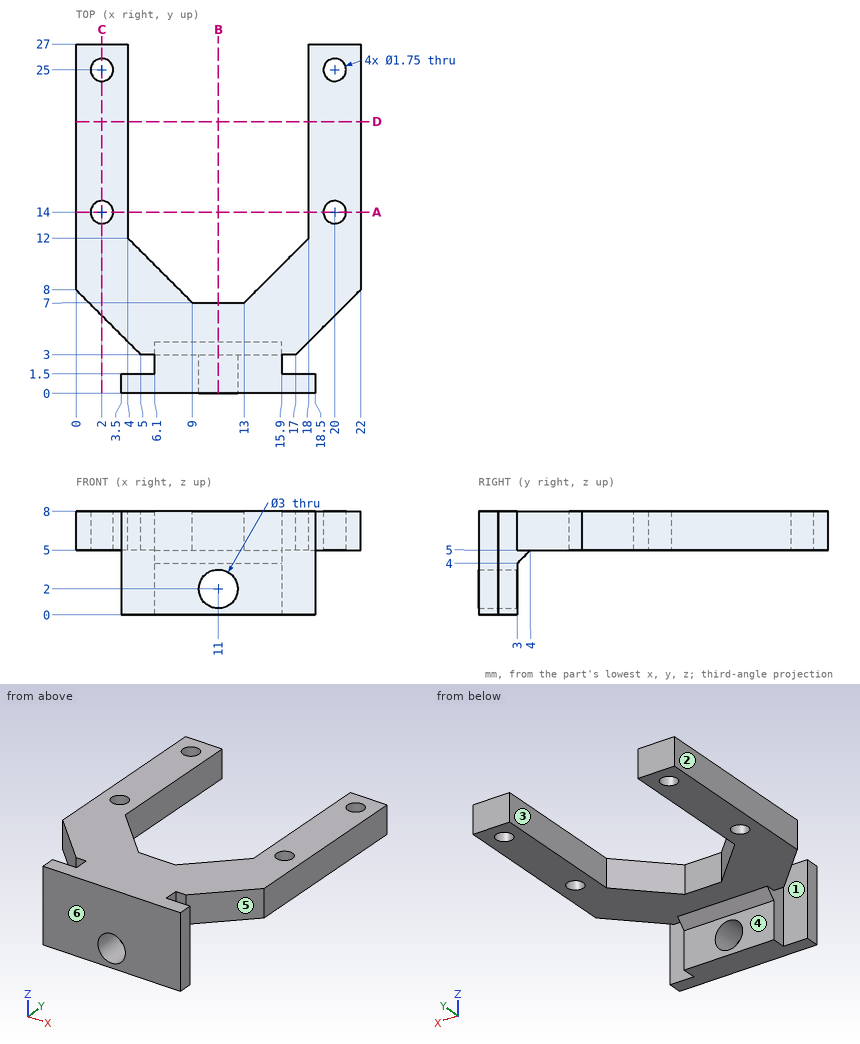
Could you check a few things on this drawing? It's one solid part, dimensions in mm from its lowest x, y, z. A direction names the side the tool comes from. Round coordinates to 2 decimals unless told otherwise and drop trailing zeros. Write each loop counter-clockwise with the first axis right and the second up, starting at its lowest first coordinate (ties: lowest second). Pieces come first, ordered by that corner, then holes.
Q1. Please list where these lines run through material, in increasing order: probe 1 along X at (y, z) = (22, 7.25); probe 2 along Y at (x, z) = (2, 6.5) (3 decimals); probe 3 along Z at (x, y) = (11, 2.2).
Q2. If we section it at D-D on y = 21: Write out the boundary of the cut face in (x, z).
Q3. Will these pins go through, and if not, where does the flat tip stop? P1, Ø1.2, axis at y = 3.5, z = 3.5, coming from the +X side; P2, Ø3, axis at y = 2.5, z = 5, coming from the -X side; P3, Ø2, axis at x = 9, z = 1, coming from the +Y side.
Q4. If we section it at B-B on x = 11: Write out the boundary of the cut face in (y, z).
Q5. If we mould it in two halves opening along Y, with no side actions, what happens to the marked faces 4, 5 and 6? For each: +Y half, -Y half, draft (parallel to the pull), parting line (faces both ways), or undercut.
Q6. If we section it at A-A on y = 14: Write out the boundary of the cut face in (x, z) (3 decimals), plus the area to 3 significant figures.
Q7. Which directions (+Z, -Z, +X, -X, +Y, -Y) give clear straight access to the entire face, cutting with the end or side of a thin tool? Please do the marked faces 1, 2 and 3.
Q8. If we section it at C-C on x = 2: Write out the boundary of the cut face in (y, z) (3 decimals), plus the area to 3 significant figures.
Answer below:
1. probe 1: x = 0 to 4, 18 to 22
1. probe 2: y = 6 to 13.125, 14.875 to 24.125, 25.875 to 27
1. probe 3: z = 0 to 0.5, 3.5 to 8
2. outline: (0, 5) - (4, 5) - (4, 8) - (0, 8) - close; (18, 5) - (22, 5) - (22, 8) - (18, 8) - close
3. P1: stops at x = 15.9
3. P2: stops at x = 3.5
3. P3: stops at y = 3
4. outline: (0, 0) - (3, 0) - (3, 0.5) - (0, 0.5) - close; (0, 3.5) - (3, 3.5) - (3, 4) - (4, 5) - (7, 5) - (7, 8) - (0, 8) - close
5. face 4: +Y half
5. face 5: undercut
5. face 6: -Y half
6. outline: (0, 5) - (1.125, 5) - (1.125, 8) - (0, 8) - close; (2.875, 5) - (4, 5) - (4, 8) - (2.875, 8) - close; (18, 5) - (19.125, 5) - (19.125, 8) - (18, 8) - close; (20.875, 5) - (22, 5) - (22, 8) - (20.875, 8) - close
6. area: 13.5 mm2
7. face 1: +Z, -Z, -X
7. face 2: +Z, -Z, -X, +Y, -Y
7. face 3: +Z, -Z, +Y
8. outline: (6, 5) - (13.125, 5) - (13.125, 8) - (6, 8) - close; (14.875, 5) - (24.125, 5) - (24.125, 8) - (14.875, 8) - close; (25.875, 5) - (27, 5) - (27, 8) - (25.875, 8) - close
8. area: 52.5 mm2
